Input: part model. Units: mm. Frame: model coordinates. A direction names the side the tool comes from. Round coordinates to 2 decimals unless told otherwise and drop trailing zeros. Order: outer loops, then holes, each group sorted by start corner. A loop starts at its lowest first (then second) coordinate and runs counter-clockwise, first axis right, second up. Notation, with made-up numbers: (1, -21.5) -> (22, -21.5) arc R11 ccw to (22, -3.5) -> close; hole circle Ø4 at (21.5, 84). An arc over 180 degrees is marked (long way). Use a Markdown table: item, result.
from build123d import *

# Parameters (mm, degrees)
BASE_FLANGE1_DEPTH           = 3.175
SKETCH8_W                    = 12.7
SKETCH8_H                    = 3.175
CUT_EXTRUDE2_DEPTH           = 318.51984313
SKETCH11_R                   = 3.175
CUT_EXTRUDE4_DEPTH           = 318.51984313
SKETCH21_R                   = 2.5527
CUT_EXTRUDE5_DEPTH           = 318.51984313
SKETCH23_W                   = 25.4
SKETCH23_H                   = 3.175
TAB1_DEPTH                   = 3.175
CSK_FOR_M3_SFHCS1_AT_2_COUNT = 2
CSK_FOR_M3_SFHCS1_AT_2_PITCH = 16
CSK_FOR_M3_SFHCS1_AT_3_COUNT = 2
CSK_FOR_M3_SFHCS1_AT_3_PITCH = 27.712812921
CSK_FOR_M3_SFHCS1_AT_4_COUNT = 2
CSK_FOR_M3_SFHCS1_AT_4_PITCH = 32
CSK_FOR_M3_SFHCS1_AT_5_COUNT = 2
CSK_FOR_M3_SFHCS1_AT_5_PITCH = 27.712812921
CSK_FOR_M3_SFHCS1_AT_6_COUNT = 2
CSK_FOR_M3_SFHCS1_AT_6_PITCH = 16
SKETCH27_R                   = 2.0193
CUT_EXTRUDE6_DEPTH           = 318.51984313
CUT_EXTRUDE8_DEPTH           = 318.51984313
FILLET2_R                    = 12.7
SKETCH29_R                   = 11.1125
CUT_EXTRUDE9_DEPTH           = 318.51984313
BREAK_CORNER1_START          = -3.175
BREAK_CORNER1_DEPTH          = 3.175
FILLET1_R                    = 2.54
FILLET4_R                    = 50.8
CUT_EXTRUDE10_DEPTH          = 318.51984313
FILLET5_R                    = 2.54


# Read off the part's stored shape, not the designer's step: Break-Corner1
# Sheet-metal steps are written as plain solids
with BuildPart() as part:
    # Sketch1 → Base-Flange1 (new body)
    with BuildSketch(Plane(origin=(0, 0, 0), x_dir=(0, 0, -1), z_dir=(1, 0, 0))):
        with BuildLine():
            Line((0, -87.3125), (0, 87.3125))
            Line((0, 87.3125), (-110.597916699, 87.3125))
            ThreePointArc((-110.597916699, 87.3125), (-137.538685062, 92.233926782), (-160.999479175, 106.3625))
            ThreePointArc((-160.999479175, 106.3625), (-201.559524406, 96.292756121), (-177.8, 61.9125))
            Line((-177.8, 61.9125), (-25.4, 61.9125))
            Line((-25.4, 61.9125), (-25.4, -61.9125))
            Line((-25.4, -61.9125), (-279.4, -61.9125))
            Line((-279.4, -61.9125), (-279.4, -74.6125))
            Line((-279.4, -74.6125), (-228.6, -74.6125))
            Line((-228.6, -74.6125), (-118.11, -150.8125))
            Line((-118.11, -150.8125), (-108.585, -150.8125))
            Line((-108.585, -150.8125), (-108.585, -144.4625))
            Line((-108.585, -144.4625), (-111.76, -144.4625))
            Line((-111.76, -144.4625), (-111.76, -125.4125))
            Line((-111.76, -125.4125), (-80.01, -125.4125))
            Line((-80.01, -125.4125), (-80.01, -144.4625))
            Line((-80.01, -144.4625), (-83.185, -144.4625))
            Line((-83.185, -144.4625), (-83.185, -150.8125))
            Line((-83.185, -150.8125), (-73.66, -150.8125))
            Line((-73.66, -150.8125), (-73.66, -100.0125))
            ThreePointArc((-73.66, -100.0125), (-69.940256121, -91.032243879), (-60.96, -87.3125))
            Line((-60.96, -87.3125), (0, -87.3125))
        make_face()
    extrude(amount=-BASE_FLANGE1_DEPTH)

    # Sketch8 → Cut-Extrude2 (cut, through all)
    with BuildSketch(Plane(origin=(0, 0, 0), x_dir=(0, 0, -1), z_dir=(1, 0, 0))):
        with Locations((-19.05, 14.2875)):
            Rectangle(SKETCH8_W, SKETCH8_H)
        with Locations((-19.05, -14.2875)):
            Rectangle(SKETCH8_W, SKETCH8_H)
    extrude(amount=-CUT_EXTRUDE2_DEPTH, mode=Mode.SUBTRACT)

    # Sketch11 → Cut-Extrude4 (cut, through all)
    with BuildSketch(Plane(origin=(0, 0, 0), x_dir=(0, 0, -1), z_dir=(1, 0, 0))):
        with Locations((-177.8, 87.3125)):
            Circle(SKETCH11_R)
    extrude(amount=-CUT_EXTRUDE4_DEPTH, mode=Mode.SUBTRACT)

    # Sketch21 → Cut-Extrude5 (cut, through all)
    with BuildSketch(Plane(origin=(0, 0, 0), x_dir=(0, 0, -1), z_dir=(1, 0, 0))):
        with Locations((-33.02, -68.2625)):
            Circle(SKETCH21_R)
        with Locations((-106.68, -68.2625)):
            Circle(SKETCH21_R)
        with Locations((-180.34, -68.2625)):
            Circle(SKETCH21_R)
        with Locations((-254, -68.2625)):
            Circle(SKETCH21_R)
        with Locations((-25.4, 68.2625)):
            Circle(SKETCH21_R)
        with Locations((-76.2, 68.2625)):
            Circle(SKETCH21_R)
        with Locations((-127, 68.2625)):
            Circle(SKETCH21_R)
    extrude(amount=-CUT_EXTRUDE5_DEPTH, mode=Mode.SUBTRACT)

    # Sketch23 → Tab1 (add)
    with BuildSketch(Plane(origin=(0, 0, 0), x_dir=(0, 0, -1), z_dir=(1, 0, 0))):
        with Locations((-217.17, -60.325)):
            Rectangle(SKETCH23_W, SKETCH23_H)
        with Locations((-143.51, -60.325)):
            Rectangle(SKETCH23_W, SKETCH23_H)
        with Locations((-69.85, -60.325)):
            Rectangle(SKETCH23_W, SKETCH23_H)
    extrude(amount=-TAB1_DEPTH)

    # Sketch25 → CSK for M3 SFHCS1 (revolve, cut)
    with BuildSketch(Plane(origin=(0, 87.3125, 161.8), x_dir=(0, 0, -1), z_dir=(0, 1, 0))):
        Polygon((0, 0), (0, 3.175), (1.7, 3.175), (1.7, 1.66), (3.36, 0), align=None)
    csk_for_m3_sfhcs1 = revolve(axis=Axis((6.35, 87.3125, 161.8), (-1, 0, 0)), mode=Mode.SUBTRACT)

    # CSK for M3 SFHCS1 at 2: CSK for M3 SFHCS1 ×2
    with Locations(*[Vector(0, -0.8660254037844383, 0.5000000000000007) * (i * CSK_FOR_M3_SFHCS1_AT_2_PITCH) for i in range(1, CSK_FOR_M3_SFHCS1_AT_2_COUNT)]):
        add(csk_for_m3_sfhcs1, mode=Mode.SUBTRACT)

    # CSK for M3 SFHCS1 at 3: CSK for M3 SFHCS1 ×2
    with Locations(*[Vector(0, -0.5000000000000007, 0.8660254037844384) * (i * CSK_FOR_M3_SFHCS1_AT_3_PITCH) for i in range(1, CSK_FOR_M3_SFHCS1_AT_3_COUNT)]):
        add(csk_for_m3_sfhcs1, mode=Mode.SUBTRACT)

    # CSK for M3 SFHCS1 at 4: CSK for M3 SFHCS1 ×2
    with Locations(*[(0, 0, i * CSK_FOR_M3_SFHCS1_AT_4_PITCH) for i in range(1, CSK_FOR_M3_SFHCS1_AT_4_COUNT)]):
        add(csk_for_m3_sfhcs1, mode=Mode.SUBTRACT)

    # CSK for M3 SFHCS1 at 5: CSK for M3 SFHCS1 ×2
    with Locations(*[Vector(0, 0.500000000000001, 0.866025403784438) * (i * CSK_FOR_M3_SFHCS1_AT_5_PITCH) for i in range(1, CSK_FOR_M3_SFHCS1_AT_5_COUNT)]):
        add(csk_for_m3_sfhcs1, mode=Mode.SUBTRACT)

    # CSK for M3 SFHCS1 at 6: CSK for M3 SFHCS1 ×2
    with Locations(*[Vector(0, 0.8660254037844392, 0.49999999999999917) * (i * CSK_FOR_M3_SFHCS1_AT_6_PITCH) for i in range(1, CSK_FOR_M3_SFHCS1_AT_6_COUNT)]):
        add(csk_for_m3_sfhcs1, mode=Mode.SUBTRACT)

    # Sketch27 → Cut-Extrude6 (cut, through all)
    with BuildSketch(Plane(origin=(0, 0, 0), x_dir=(0, 0, -1), z_dir=(1, 0, 0))):
        with Locations((-85.09, -93.6625)):
            Circle(SKETCH27_R)
        with Locations(Location((-85.09, -112.7125, 0), (0, 0, 180))):
            Circle(SKETCH27_R)
        with Locations((-106.68, -112.7125)):
            Circle(SKETCH27_R)
        with Locations(Location((-106.68, -93.6625, 0), (0, 0, 180))):
            Circle(SKETCH27_R)
        with BuildLine():
            Line((-107.442, -98.45675), (-102.106618912, -98.45675))
            ThreePointArc((-102.106618912, -98.45675), (-101.283564844, -98.658721447), (-100.6475, -99.21875))
            Line((-100.6475, -99.21875), (-91.1225, -99.21875))
            ThreePointArc((-91.1225, -99.21875), (-90.486435156, -98.658721447), (-89.663381088, -98.45675))
            Line((-89.663381088, -98.45675), (-84.328, -98.45675))
            ThreePointArc((-84.328, -98.45675), (-83.070764143, -98.977514143), (-82.55, -100.23475))
            Line((-82.55, -100.23475), (-82.55, -106.14025))
            ThreePointArc((-82.55, -106.14025), (-83.070764143, -107.397485857), (-84.328, -107.91825))
            Line((-84.328, -107.91825), (-89.663381088, -107.91825))
            ThreePointArc((-89.663381088, -107.91825), (-90.486435156, -107.716278553), (-91.1225, -107.15625))
            Line((-91.1225, -107.15625), (-100.6475, -107.15625))
            ThreePointArc((-100.6475, -107.15625), (-101.283564844, -107.716278553), (-102.106618912, -107.91825))
            Line((-102.106618912, -107.91825), (-107.442, -107.91825))
            ThreePointArc((-107.442, -107.91825), (-108.699235857, -107.397485857), (-109.22, -106.14025))
            Line((-109.22, -106.14025), (-109.22, -100.23475))
            ThreePointArc((-109.22, -100.23475), (-108.699235857, -98.977514143), (-107.442, -98.45675))
        make_face()
    extrude(amount=-CUT_EXTRUDE6_DEPTH, mode=Mode.SUBTRACT)

    # Sketch28 → Cut-Extrude8 (cut, through all)
    with BuildSketch(Plane(origin=(0, 0, 0), x_dir=(0, 0, -1), z_dir=(1, 0, 0))):
        with BuildLine():
            Line((-111.76, -144.4625), (-111.76, -141.1605))
            ThreePointArc((-111.76, -141.1605), (-113.411, -142.8115), (-111.76, -144.4625))
        make_face()
        with BuildLine():
            Line((-80.01, -144.4625), (-80.01, -141.1605))
            ThreePointArc((-80.01, -141.1605), (-78.359, -142.8115), (-80.01, -144.4625))
        make_face()
        with BuildLine():
            Line((-80.01, -125.4125), (-80.01, -128.7145))
            ThreePointArc((-80.01, -128.7145), (-78.359, -127.0635), (-80.01, -125.4125))
        make_face()
        with BuildLine():
            Line((-111.76, -125.4125), (-111.76, -128.7145))
            ThreePointArc((-111.76, -128.7145), (-113.411, -127.0635), (-111.76, -125.4125))
        make_face()
        with BuildLine():
            ThreePointArc((-15.458644321, -14.2875), (-14.298573876, -17.11325), (-13.138503431, -14.2875))
            ThreePointArc((-13.138503431, -14.2875), (-14.298573876, -11.46175), (-15.458644321, -14.2875))
        make_face()
        with BuildLine():
            ThreePointArc((-15.458644321, 14.2875), (-14.298573876, 11.46175), (-13.138503431, 14.2875))
            ThreePointArc((-13.138503431, 14.2875), (-14.298573876, 17.11325), (-15.458644321, 14.2875))
        make_face()
    extrude(amount=-CUT_EXTRUDE8_DEPTH, mode=Mode.SUBTRACT)

    # Fillet2
    fillet2_edges = [part.edges().sort_by_distance(p)[0] for p in [
        (-1.5875, -87.3125, 0),
        (-1.5875, -150.8125, 118.11),
    ]]
    fillet(fillet2_edges, radius=FILLET2_R)

    # Sketch29 → Cut-Extrude9 (cut, through all)
    with BuildSketch(Plane.ZY.offset(3.175)):
        with Locations((177.8, 87.3125)):
            Circle(SKETCH29_R)
    extrude(amount=-CUT_EXTRUDE9_DEPTH, mode=Mode.SUBTRACT)

    # Break-Corner1 outline → Break-Corner1 (cut)
    with BuildSketch(Plane.YZ.offset(BREAK_CORNER1_START)):
        with BuildLine():
            ThreePointArc((87.3125, 12.7), (83.592756121, 3.719743879), (74.6125, 0))
            Line((74.6125, 0), (87.3125, 0))
            Line((87.3125, 0), (87.3125, 12.7))
        make_face()
    extrude(amount=BREAK_CORNER1_DEPTH, mode=Mode.SUBTRACT)

    # Fillet1
    fillet1_edges = [part.edges().sort_by_distance(p)[0] for p in [
        (-1.5875, -61.9125, 229.87),
        (-1.5875, -61.9125, 204.47),
        (-1.5875, -61.9125, 156.21),
        (-1.5875, -61.9125, 130.81),
        (-1.5875, -61.9125, 82.55),
        (-1.5875, -61.9125, 57.15),
        (-1.5875, -150.8125, 73.66),
        (-1.5875, -150.8125, 83.185),
        (-1.5875, -150.8125, 108.585),
        (-1.5875, -74.6125, 279.4),
        (-1.5875, -61.9125, 279.4),
        (-1.5875, -61.9125, 25.4),
        (-1.5875, 61.9125, 25.4),
    ]]
    fillet(fillet1_edges, radius=FILLET1_R)

    # Fillet4
    fillet4_edges = [part.edges().sort_by_distance(p)[0] for p in [
        (-1.5875, -74.6125, 228.6),
    ]]
    fillet(fillet4_edges, radius=FILLET4_R)

    # Sketch30 → Cut-Extrude10 (cut, through all)
    with BuildSketch(Plane.ZY.offset(3.175)):
        Polygon((124.46, -134.86266966), (163.882081016, -107.67502758), (124.46, -82.654490572), align=None)
        Polygon((211.822746006, -74.6125), (129.564117224, -74.6125), (172.400664991, -101.80014208), align=None)
    extrude(amount=-CUT_EXTRUDE10_DEPTH, mode=Mode.SUBTRACT)

    # Fillet5
    fillet5_edges = [part.edges().sort_by_distance(p)[0] for p in [
        (-1.5875, -74.6125, 211.822746006),
        (-1.5875, -101.80014208, 172.400664991),
        (-1.5875, -74.6125, 129.564117224),
        (-1.5875, -134.86266966, 124.46),
        (-1.5875, -82.654490572, 124.46),
        (-1.5875, -107.67502758, 163.882081016),
    ]]
    fillet(fillet5_edges, radius=FILLET5_R)


solid = part.part
1) Line query: L1, parallel to Y at x = -0.95, z = 106.68; L2, parallel to Y at x = -2.4, z = 33.02; L3, parallel to Z at x = -1.65, y = -66.5. Output: solid intervals per line, ascending. Write a range as [from, to].
Results found:
| item | result |
|---|---|
| L1 | y = [-125.41, -114.73], [-110.69, -107.92], [-98.46, -95.68], [-91.64, -70.82], [-65.71, -61.91], [61.91, 87.31] |
| L2 | y = [-87.31, -70.82], [-65.71, -61.91], [61.91, 87.31] |
| L3 | z = [0, 31.17], [34.87, 104.83], [108.53, 178.49], [182.19, 252.15], [255.85, 279.4] |
2) Set-up query: faces 1 (the flat face through (0, -67, 89)), 2 (the flat face through (-1.61, -90.196, 189.227)). Return all of +Z, -Z, +X, -X, +Y, -Y with unobstructed straight access to the full face (end or side cutting, diameter ignored); none if empty.
Results found:
| item | result |
|---|---|
| face 1 | +Z, -Z, +X, +Y, -Y |
| face 2 | +X, -X |
3) Cut plane B-B on y = 35. Return loops of the section in (x, z) (3 decimals).
Results found:
| item | result |
|---|---|
| outline | (-3.175, 0) -> (0, 0) -> (0, 25.4) -> (-3.175, 25.4) -> close |
4) Pin query (flat end, axial travel): pin 1 Ø1.6 at (x, z) = (-1, 86.5) entering from +Y; pin 2 Ø1 at (x, z) = (-1.5, 189.5) entering from +Y; pin 3 Ø1.6 at (x, y) = (-1.5, -103.5) entering from +Z. Return the tip coordinate at first contact, or that it passes through.
Results found:
| item | result |
|---|---|
| pin 1 | stops at y = 87.31 |
| pin 2 | stops at y = 110.11 |
| pin 3 | stops at z = 187.87 |
5) Pull-direction query (Z, two-part tool) for faces 3 (the cylindrical face through (-1.61, 83.056, 188.065)), 4 (the flat face through (-3.175, -67, 78)), 5 (the flat face through (-1.61, -121.14, 144.36)), 6 (the cylindrical face through (-1.565, -91.132, 70.038)); classes: +Z half, -Z half, draft (parallel to the pull), parting line (faces both ways), or undercut.
Results found:
| item | result |
|---|---|
| face 3 | undercut |
| face 4 | draft |
| face 5 | undercut |
| face 6 | -Z half |
6) Cut plane A-A on x = -0.65. Count the separate pieces of the cut face and the enclosed holes in it, and give its area (3 significant figures).
Results found:
| item | result |
|---|---|
| separate pieces | 1 |
| enclosed holes | 21 |
| area | 17,700 mm² |
